Autodesk Fusion 360 part; units mm, degrees
sketch "スケッチ1" plane through (0, 0, 0) normal (0, 0, 1) x (1, 0, 0)
  line L0 (65.6268, -79.7784) -> (8.6268, -79.7784)
  line L1 (8.6268, -75.2784) -> (65.6268, -75.2784)
  line L2 (8.6268, 65.7216) -> (65.6268, 65.7216)
  line L3 (8.6268, 70.2216) -> (65.6268, 70.2216)
  line L4 (4.1268, 61.2216) -> (4.1268, -70.7784)
  line L5 (-0.3732, 61.2216) -> (-0.3732, -70.7784)
  arc A0 (-0.3732, -70.7784) -> (8.6268, -79.7784) centre (8.6268, -70.7784) ccw
  arc A1 (4.1268, -70.7784) -> (8.6268, -75.2784) centre (8.6268, -70.7784) ccw
  arc A2 (8.6268, 70.2216) -> (-0.3732, 61.2216) centre (8.6268, 61.2216) ccw
  arc A3 (8.6268, 65.7216) -> (4.1268, 61.2216) centre (8.6268, 61.2216) ccw
  line L6 (70.1268, -70.7784) -> (70.1268, -54.7784)
  line L7 (74.6268, -70.7784) -> (74.6268, -54.7784)
  arc A4 (65.6268, -79.7784) -> (74.6268, -70.7784) centre (65.6268, -70.7784) ccw
  arc A5 (65.6268, -75.2784) -> (70.1268, -70.7784) centre (65.6268, -70.7784) ccw
  line L8 (74.6268, -54.7784) -> (70.1268, -54.7784)
  line L9 (74.6268, 61.2216) -> (74.6268, 45.2216)
  line L10 (70.1268, 61.2216) -> (70.1268, 45.2216)
  line L11 (70.1268, 45.2216) -> (74.6268, 45.2216)
  arc A6 (74.6268, 61.2216) -> (65.6268, 70.2216) centre (65.6268, 61.2216) ccw
  arc A7 (70.1268, 61.2216) -> (65.6268, 65.7216) centre (65.6268, 61.2216) ccw
  point P0 (-0.3732, 70.2216)
extrude "押し出し1" add sketch "スケッチ1" along normal blind 100
Can you work these out from the model? Positions are in its coordinate system, mm. A direction names the side the tool comes from. Give positions to 0.01 mm unless a question says otherwise; leave off trailing zeros. Write each loop counter-clockwise with the first axis right and the second up, starting at its lowest first coordinate (ties: lowest second). Pieces come first, ordered by that corner, then holes. Notation, with made-up numbers: M -2,63 L 5,63 A20 cw 5,102 Z; hole C 26,20 d6. An arc over 180 degrees is marked long. Answer in a Markdown table with one row per item. Add a question column.
Item 1: Imagine slicing it at C-C, the plane z = 48.5. Write out the boundary of the cut face in (x, y), plus the area to 3 significant figures.
Item 2: Imagine slicing it at A-A, the plane x = 40.5. Write out the boundary of the cut face in (y, z).
Item 3: Imagine slicing it at D-D, the plane y = -15.5. Write out the boundary of the cut face in (x, z).
Item 4: We'd pull the mould along X, two halves only. Please class faces 3 (the cylindrical face through (5.48, -73.995, 49.3)), 4 (the flat face through (72, -54.778, 49)), 5 (the flat face through (74.627, 53, 49)): released by +X, released by -X, zero draft, split by the parting line, or undercut.
Item 5: For pin 1 Ø5 at (y, z) = (-8, 63.5) entering from +X; pin 2 Ø3.5 at (x, z) = (72.5, 55) entering from +Y; pin 3 Ø1.3 at (x, z) = (72.5, 29) entering from -Y, each with a flat end and sliding along its axis, tell me the tip position at first contact or that it passes through.
Item 6: On a 3-axis mill with a long thin cutter (end or side, diameter ignored), from which of +Z, -Z, +X, -X, +Y, -Y can I reach the whole of each face in a straight line? I mean faces 1 (the cylindrical face through (2.33, -77.21, 49.3)), 2 (the flat face through (70.127, 53, 49)). Say none if no direction works.
Item 7: Please list where these lines run through material, in increasing order: L1, parallel to Y at x = 65.5, z = 65; L2, parallel to X at y = 61.5, z = 73; L3, parallel to X at y = -5, z = 55.
Item 8: Imagine slicing it at B-B, the plane y = 50. Write out the boundary of the cut face in (x, z), plus the area to 3 significant figures.
Evaluation:
| question | item | result |
|---|---|---|
| 1 | outline | M -0.37,-70.78 A9 ccw 8.63,-79.78 L 65.63,-79.78 A9 ccw 74.63,-70.78 L 74.63,-54.78 L 70.13,-54.78 L 70.13,-70.78 A4.5 cw 65.63,-75.28 L 8.63,-75.28 A4.5 cw 4.13,-70.78 L 4.13,61.22 A4.5 cw 8.63,65.72 L 65.63,65.72 A4.5 cw 70.13,61.22 L 70.13,45.22 L 74.63,45.22 L 74.63,61.22 A9 ccw 65.63,70.22 L 8.63,70.22 A9 ccw -0.37,61.22 Z |
| 1 | area | 1,440 mm² |
| 2 | outline | M -79.78,0 L -75.28,0 L -75.28,100 L -79.78,100 Z; M 65.72,0 L 70.22,0 L 70.22,100 L 65.72,100 Z |
| 3 | outline | M -0.37,0 L 4.13,0 L 4.13,100 L -0.37,100 Z |
| 4 | face 3 | undercut |
| 4 | face 4 | zero draft |
| 4 | face 5 | released by +X |
| 5 | pin 1 | stops at x = 4.13 |
| 5 | pin 2 | stops at y = 68.62 |
| 5 | pin 3 | stops at y = -77.28 |
| 6 | face 1 | +Z, -Z, -X, -Y |
| 6 | face 2 | +Z, -Z |
| 7 | L1 | y = -79.78 to -75.28, 65.72 to 70.22 |
| 7 | L2 | x = -0.37 to 4.14, 70.12 to 74.62 |
| 7 | L3 | x = -0.37 to 4.13 |
| 8 | outline | M -0.37,0 L 4.13,0 L 4.13,100 L -0.37,100 Z; M 70.13,0 L 74.63,0 L 74.63,100 L 70.13,100 Z |
| 8 | area | 900 mm² |
